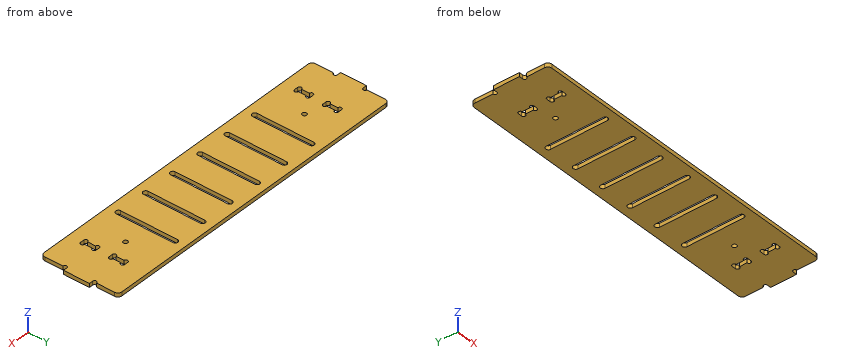
from build123d import *

# Parameters (mm, degrees)
SKETCH_1_W          = 254
SKETCH_1_H          = 55
EXTRUDE_1_DEPTH     = 3
SKETCH_2_W          = 3
SKETCH_2_H          = 20
SKETCH_2_H_2        = 15
CUT_EXTRUDE_1_DEPTH = 130.977882734
SKETCH_3_W          = 3
SKETCH_3_H          = 12
CUT_EXTRUDE_2_DEPTH = 130.977882734
CUT_EXTRUDE_3_DEPTH = 130.977882734
SKETCH_5_R          = 1.5
CUT_EXTRUDE_4_DEPTH = 130.977882734
SKETCH_6_R          = 1.7
CUT_EXTRUDE_5_DEPTH = 130.977882734
SKETCH_7_W          = 248
SKETCH_7_H          = 3
EXTRUDE_2_DEPTH     = 5
CUT_EXTRUDE_6_DEPTH = 132.126846984
FILLET_1_R          = 3


with BuildPart() as part:
    # 草图1 → 凸台-拉伸1 (new body)
    with BuildSketch(Plane.XY):
        Rectangle(SKETCH_1_W, SKETCH_1_H)
    extrude(amount=EXTRUDE_1_DEPTH)

    # 草图2 → 切除-拉伸1 (cut, through all)
    with BuildSketch(Plane.XY.offset(3)):
        with Locations((-125.5, -17.5)):
            Rectangle(SKETCH_2_W, SKETCH_2_H)
        with Locations((-125.5, 20)):
            Rectangle(SKETCH_2_W, SKETCH_2_H_2)
        with Locations((125.5, -17.5)):
            Rectangle(SKETCH_2_W, SKETCH_2_H)
        with Locations((125.5, 20)):
            Rectangle(SKETCH_2_W, SKETCH_2_H_2)
    extrude(amount=-CUT_EXTRUDE_1_DEPTH, mode=Mode.SUBTRACT)

    # 草图3 → 切除-拉伸2 (cut, through all)
    with BuildSketch(Plane.XY.offset(3)):
        with Locations((-98, -11.5)):
            Rectangle(SKETCH_3_W, SKETCH_3_H)
        with Locations((-98, 10.5)):
            Rectangle(SKETCH_3_W, SKETCH_3_H)
        with Locations((98, -11.5)):
            Rectangle(SKETCH_3_W, SKETCH_3_H)
        with Locations((98, 10.5)):
            Rectangle(SKETCH_3_W, SKETCH_3_H)
    extrude(amount=-CUT_EXTRUDE_2_DEPTH, mode=Mode.SUBTRACT)

    # 草图4 → 切除-拉伸3 (cut, through all)
    with BuildSketch(Plane.XY.offset(3)):
        with BuildLine():
            Line((99.5, -14.5), (99.5, -17.5))
            ThreePointArc((99.5, -17.5), (100.560660172, -17.060660172), (101, -16))
            ThreePointArc((101, -16), (100.560660172, -14.939339828), (99.5, -14.5))
        make_face()
        with BuildLine():
            ThreePointArc((99.5, -14.5), (98, -16), (99.5, -17.5))
            Line((99.5, -17.5), (99.5, -14.5))
        make_face()
        with BuildLine():
            Line((96.5, -14.55), (96.5, -17.5))
            ThreePointArc((96.5, -17.5), (97.542982502, -17.067982502), (97.975, -16.025))
            ThreePointArc((97.975, -16.025), (97.542982502, -14.982017498), (96.5, -14.55))
        make_face()
        with BuildLine():
            ThreePointArc((96.5, -14.55), (95.025, -16.025), (96.5, -17.5))
            Line((96.5, -17.5), (96.5, -14.55))
        make_face()
        with BuildLine():
            ThreePointArc((96.5, -5.5), (95.025, -6.975), (96.5, -8.45))
            Line((96.5, -8.45), (96.5, -5.5))
        make_face()
        with BuildLine():
            Line((96.5, -5.5), (96.5, -8.45))
            ThreePointArc((96.5, -8.45), (97.542982502, -8.017982502), (97.975, -6.975))
            ThreePointArc((97.975, -6.975), (97.542982502, -5.932017498), (96.5, -5.5))
        make_face()
        with BuildLine():
            ThreePointArc((99.5, -5.5), (98, -7), (99.5, -8.5))
            Line((99.5, -8.5), (99.5, -5.5))
        make_face()
        with BuildLine():
            Line((99.5, -5.5), (99.5, -8.5))
            ThreePointArc((99.5, -8.5), (100.560660172, -8.060660172), (101, -7))
            ThreePointArc((101, -7), (100.560660172, -5.939339828), (99.5, -5.5))
        make_face()
        with BuildLine():
            ThreePointArc((99.5, 7.5), (98.439339828, 7.060660172), (98, 6))
            ThreePointArc((98, 6), (98.439339828, 4.939339828), (99.5, 4.5))
            Line((99.5, 4.5), (99.5, 7.5))
        make_face()
        with BuildLine():
            Line((99.5, 7.5), (99.5, 4.5))
            ThreePointArc((99.5, 4.5), (100.560660172, 4.939339828), (101, 6))
            ThreePointArc((101, 6), (100.560660172, 7.060660172), (99.5, 7.5))
        make_face()
        with BuildLine():
            Line((96.5, 7.5), (96.5, 4.5))
            ThreePointArc((96.5, 4.5), (97.560660172, 4.939339828), (98, 6))
            ThreePointArc((98, 6), (97.560660172, 7.060660172), (96.5, 7.5))
        make_face()
        with BuildLine():
            ThreePointArc((96.5, 7.5), (95, 6), (96.5, 4.5))
            Line((96.5, 4.5), (96.5, 7.5))
        make_face()
        with BuildLine():
            Line((96.5, 16.5), (96.5, 13.5))
            ThreePointArc((96.5, 13.5), (97.560660172, 13.939339828), (98, 15))
            ThreePointArc((98, 15), (97.560660172, 16.060660172), (96.5, 16.5))
        make_face()
        with BuildLine():
            ThreePointArc((96.5, 16.5), (95, 15), (96.5, 13.5))
            Line((96.5, 13.5), (96.5, 16.5))
        make_face()
        with BuildLine():
            Line((99.5, 16.5), (99.5, 13.5))
            ThreePointArc((99.5, 13.5), (100.560660172, 13.939339828), (101, 15))
            ThreePointArc((101, 15), (100.560660172, 16.060660172), (99.5, 16.5))
        make_face()
        with BuildLine():
            ThreePointArc((98, 15), (98.439339828, 13.939339828), (99.5, 13.5))
            Line((99.5, 13.5), (99.5, 16.5))
            ThreePointArc((99.5, 16.5), (98.439339828, 16.060660172), (98, 15))
        make_face()
        with BuildLine():
            ThreePointArc((-96.5, 13.5), (-95.439339828, 13.939339828), (-95, 15))
            ThreePointArc((-95, 15), (-95.439339828, 16.060660172), (-96.5, 16.5))
            Line((-96.5, 16.5), (-96.5, 13.5))
        make_face()
        with BuildLine():
            Line((-96.5, 13.5), (-96.5, 16.5))
            ThreePointArc((-96.5, 16.5), (-97.560660172, 16.060660172), (-98, 15))
            ThreePointArc((-98, 15), (-97.560660172, 13.939339828), (-96.5, 13.5))
        make_face()
        with BuildLine():
            ThreePointArc((-99.5, 13.5), (-98.439339828, 13.939339828), (-98, 15))
            ThreePointArc((-98, 15), (-98.439339828, 16.060660172), (-99.5, 16.5))
            Line((-99.5, 16.5), (-99.5, 13.5))
        make_face()
        with BuildLine():
            Line((-99.5, 13.5), (-99.5, 16.5))
            ThreePointArc((-99.5, 16.5), (-101, 15), (-99.5, 13.5))
        make_face()
        with BuildLine():
            ThreePointArc((-99.5, 4.5), (-98.439339828, 4.939339828), (-98, 6))
            ThreePointArc((-98, 6), (-98.439339828, 7.060660172), (-99.5, 7.5))
            Line((-99.5, 7.5), (-99.5, 4.5))
        make_face()
        with BuildLine():
            Line((-99.5, 4.5), (-99.5, 7.5))
            ThreePointArc((-99.5, 7.5), (-101, 6), (-99.5, 4.5))
        make_face()
        with BuildLine():
            Line((-96.5, 4.5), (-96.5, 7.5))
            ThreePointArc((-96.5, 7.5), (-97.560660172, 7.060660172), (-98, 6))
            ThreePointArc((-98, 6), (-97.560660172, 4.939339828), (-96.5, 4.5))
        make_face()
        with BuildLine():
            ThreePointArc((-95, 6), (-95.439339828, 7.060660172), (-96.5, 7.5))
            Line((-96.5, 7.5), (-96.5, 4.5))
            ThreePointArc((-96.5, 4.5), (-95.439339828, 4.939339828), (-95, 6))
        make_face()
        with BuildLine():
            ThreePointArc((-96.5, -8.45), (-95.457017498, -8.017982502), (-95.025, -6.975))
            ThreePointArc((-95.025, -6.975), (-95.457017498, -5.932017498), (-96.5, -5.5))
            Line((-96.5, -5.5), (-96.5, -8.45))
        make_face()
        with BuildLine():
            Line((-96.5, -8.45), (-96.5, -5.5))
            ThreePointArc((-96.5, -5.5), (-97.975, -6.975), (-96.5, -8.45))
        make_face()
        with BuildLine():
            ThreePointArc((-99.5, -8.5), (-98.439339828, -8.060660172), (-98, -7))
            ThreePointArc((-98, -7), (-98.439339828, -5.939339828), (-99.5, -5.5))
            Line((-99.5, -5.5), (-99.5, -8.5))
        make_face()
        with BuildLine():
            Line((-99.5, -8.5), (-99.5, -5.5))
            ThreePointArc((-99.5, -5.5), (-101, -7), (-99.5, -8.5))
        make_face()
        with BuildLine():
            ThreePointArc((-98, -16), (-98.439339828, -14.939339828), (-99.5, -14.5))
            Line((-99.5, -14.5), (-99.5, -17.5))
            ThreePointArc((-99.5, -17.5), (-98.439339828, -17.060660172), (-98, -16))
        make_face()
        with BuildLine():
            Line((-99.5, -17.5), (-99.5, -14.5))
            ThreePointArc((-99.5, -14.5), (-101, -16), (-99.5, -17.5))
        make_face()
        with BuildLine():
            ThreePointArc((-95.025, -16.025), (-95.457017498, -14.982017498), (-96.5, -14.55))
            Line((-96.5, -14.55), (-96.5, -17.5))
            ThreePointArc((-96.5, -17.5), (-95.457017498, -17.067982502), (-95.025, -16.025))
        make_face()
        with BuildLine():
            Line((-96.5, -17.5), (-96.5, -14.55))
            ThreePointArc((-96.5, -14.55), (-97.975, -16.025), (-96.5, -17.5))
        make_face()
    extrude(amount=-CUT_EXTRUDE_3_DEPTH, mode=Mode.SUBTRACT)

    # 草图5 → 切除-拉伸4 (cut, through all)
    with BuildSketch(Plane.XY.offset(3)):
        with Locations((-124, 14)):
            Circle(SKETCH_5_R)
        with Locations((-124, -9)):
            Circle(SKETCH_5_R)
        with Locations((124, -9)):
            Circle(SKETCH_5_R)
        with Locations((124, 14)):
            Circle(SKETCH_5_R)
    extrude(amount=-CUT_EXTRUDE_4_DEPTH, mode=Mode.SUBTRACT)

    # 草图6 → 切除-拉伸5 (cut, through all)
    with BuildSketch(Plane.XY.offset(3)):
        with Locations((-82, 2.5)):
            Circle(SKETCH_6_R)
        with Locations(Location((82, 2.5, 0), (0, 0, 180))):
            Circle(SKETCH_6_R)
    extrude(amount=-CUT_EXTRUDE_5_DEPTH, mode=Mode.SUBTRACT)

    # 草图7 → 凸台-拉伸2 (add)
    with BuildSketch(Plane(origin=(0, 27.5, 0), x_dir=(1, 0, 0), z_dir=(0, 1, 0))):
        with Locations((0, -1.5)):
            Rectangle(SKETCH_7_W, SKETCH_7_H)
    extrude(amount=EXTRUDE_2_DEPTH)

    # 草图8 → 切除-拉伸6 (cut, through all)
    with BuildSketch(Plane.XY.offset(3)):
        with BuildLine():
            Line((-60.5, 24.5), (-60.5, -19.5))
            ThreePointArc((-60.5, -19.5), (-62.5, -21.5), (-64.5, -19.5))
            Line((-64.5, -19.5), (-64.5, 24.5))
            ThreePointArc((-64.5, 24.5), (-62.5, 26.5), (-60.5, 24.5))
        make_face()
        with BuildLine():
            Line((-39.5, 24.5), (-39.5, -19.5))
            ThreePointArc((-39.5, -19.5), (-37.5, -21.5), (-35.5, -19.5))
            Line((-35.5, -19.5), (-35.5, 24.5))
            ThreePointArc((-35.5, 24.5), (-37.5, 26.5), (-39.5, 24.5))
        make_face()
        with BuildLine():
            Line((-14.5, 24.5), (-14.5, -19.5))
            ThreePointArc((-14.5, -19.5), (-12.5, -21.5), (-10.5, -19.5))
            Line((-10.5, -19.5), (-10.5, 24.5))
            ThreePointArc((-10.5, 24.5), (-12.5, 26.5), (-14.5, 24.5))
        make_face()
        with BuildLine():
            Line((60.5, 24.5), (60.5, -19.5))
            ThreePointArc((60.5, -19.5), (62.5, -21.5), (64.5, -19.5))
            Line((64.5, -19.5), (64.5, 24.5))
            ThreePointArc((64.5, 24.5), (62.5, 26.5), (60.5, 24.5))
        make_face()
        with BuildLine():
            Line((35.5, 24.5), (35.5, -19.5))
            ThreePointArc((35.5, -19.5), (37.5, -21.5), (39.5, -19.5))
            Line((39.5, -19.5), (39.5, 24.5))
            ThreePointArc((39.5, 24.5), (37.5, 26.5), (35.5, 24.5))
        make_face()
        with BuildLine():
            Line((10.5, 24.5), (10.5, -19.5))
            ThreePointArc((10.5, -19.5), (12.5, -21.5), (14.5, -19.5))
            Line((14.5, -19.5), (14.5, 24.5))
            ThreePointArc((14.5, 24.5), (12.5, 26.5), (10.5, 24.5))
        make_face()
    extrude(amount=-CUT_EXTRUDE_6_DEPTH, mode=Mode.SUBTRACT)

    # 圆角1
    fillet_1_edges = [part.edges().sort_by_distance(p)[0] for p in [
        (124, 32.5, 1.5),
        (-124, 32.5, 1.5),
        (124, -27.5, 1.5),
        (-124, -27.5, 1.5),
    ]]
    fillet(fillet_1_edges, radius=FILLET_1_R)


solid = part.part
Check sheet for the modelled part. Datum: model origin and axes. Units: mm. Round coordinates to 2 decimals unless told otherwise and drop trailing zeros. Order: outer loops, then holes, each group sorted by start corner. A loop starts at its lowest first (then second) coordinate and runs counter-clockwise, first axis right, second up.
(1) Go/stop test with flat-tipped pins: P1, Ø0.9, axis at y = 22.5, z = 1.5, coming from the +X side; P2, Ø10, axis at x = -38.5, y = 25.5, coming from the -Z side. Record where each tip stops, or that it passes through.
(2) Cross-section at A-A, the plane y = 21. Enter the section's corners in (x, z), and give its area (3 significant figures).
(3) Cross-section at B-B, the plane z = 0.95. State how many separate pieces and enclosed holes the cut face has, and give its area (3 significant figures).
(4) Scan lines: probe 1 along Y at (x, z) = (-82, 1.3); probe 2 along Y at (x, z) = (-63.5, 0.95); probe 3 along X at (y, z) = (-22, 1.1). Record each from-to range of solid material in increasing order.
Check sheet entries:
1. P1: stops at x = 124
1. P2: stops at z = 0
2. outline: (-124, 0) - (-64.5, 0) - (-64.5, 3) - (-124, 3) - close; (-60.5, 0) - (-39.5, 0) - (-39.5, 3) - (-60.5, 3) - close; (-35.5, 0) - (-14.5, 0) - (-14.5, 3) - (-35.5, 3) - close; (-10.5, 0) - (10.5, 0) - (10.5, 3) - (-10.5, 3) - close; (14.5, 0) - (35.5, 0) - (35.5, 3) - (14.5, 3) - close; (39.5, 0) - (60.5, 0) - (60.5, 3) - (39.5, 3) - close; (64.5, 0) - (124, 0) - (124, 3) - (64.5, 3) - close
2. area: 672 mm2
3. separate pieces: 1
3. enclosed holes: 12
3. area: 13,600 mm2
4. probe 1: y = -27.5 to 0.8, 4.2 to 32.5
4. probe 2: y = -27.5 to -21.23, 26.23 to 32.5
4. probe 3: x = -124 to 124
